Design review of the part built by this model. Coordinates are the model's own, in mm. Give positions to 0.01 mm unless a question says otherwise; leave off trailing zeros. Loops run counter-clockwise (first coordinate to the right, second up) from the corner with the lowest first, then second, coordinate; pieces in that order, holes last. Notation, with made-up numbers: M -25.75,1.5 L 9.25,1.5 A25 ccw 9.25,19.5 Z; hole C 13,7 d9. An arc over 180 degrees is marked long. Use one line per item in the form item = value. Start each with the question number.
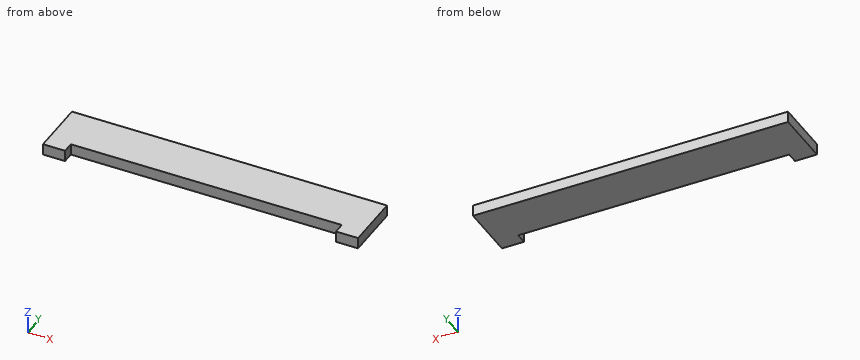
Autodesk Inventor part; units mm, degrees
ref_plane "YZ Plane" through (0, 0, 0) normal (1, 0, 0) x (0, 1, 0)
ref_plane "XZ Plane" through (0, 0, 0) normal (0, 1, 0) x (-1, 0, 0)
ref_plane "XY Plane" through (0, 0, 0) normal (0, 0, 1) x (1, 0, 0)
sketch "Sketch1" plane through (0, 0, 0) normal (0, 0, 1) x (1, 0, 0)
  line L0 (-70, -10) -> (70, -10)
  line L1 (70, -10) -> (70, 10)
  line L2 (70, 10) -> (-70, 10)
  line L3 (-70, 10) -> (-70, -10)
  point P0 (0, 0)
  dimension "width" = 140
  dimension "d1" = 70
  dimension "d2" = 20
  dimension "d3" = 10
extrude "Extrusion1" add sketch "Sketch1" along normal blind 5
sketch "Sketch3" plane through (-70, -10, 0) normal (0, -1, 0) x (1, 0, 0)
  line L0 (0, 0) -> (140, 0)
  line L1 (0, 5) -> (140, 5)
  line L2 (0, 0) -> (9.8, 0)
  line L3 (9.8, 0) -> (9.8, 5)
  line L4 (9.8, 5) -> (0, 5)
  line L5 (0, 5) -> (0, 0)
  point P0 (70, 0)
  dimension "d28" = 9.8
extrude "Extrusion3" add sketch "Sketch3" along normal blind 5
mirror "Mirror1" about plane through (0, 0, 0) normal (1, 0, 0) of "Extrusion3"
properties part number "EBF_004.1-back-plate_cup-holder"
Q1. Wall thickness on probe 1 along X at (y, z) = (-12.5, 4.25); probe 2 along Y at (x, z) = (13, 2.2): over which ranges is each line inside the solid? List them lowest first.
Q2. Take a section at B-B on x = -2.5. Give the boundary of the cut face in (y, z).
Q3. Take a section at A-A on z = 3.5. Give the boundary of the cut face in (x, y), plus the area to 3 significant figures.
Q4. Clearance check with flat-ended pins moving along their axes: pin 1 Ø5 at (x, y) = (-49, -2) entering from -Z; pin 2 Ø1.5 at (x, z) = (15.5, 1.5) entering from -Y. State where each tip first meets the part, or that it passes through.
Response values:
q1.probe_1 = -70 to -60.2, 60.2 to 70
q1.probe_2 = -10 to 10
q2.outline = M -10,0 L 10,0 L 10,5 L -10,5 Z
q3.outline = M -70,-15 L -60.2,-15 L -60.2,-10 L 60.2,-10 L 60.2,-15 L 70,-15 L 70,10 L -70,10 Z
q3.area = 2,900 mm^2
q4.pin_1 = 0
q4.pin_2 = -10
